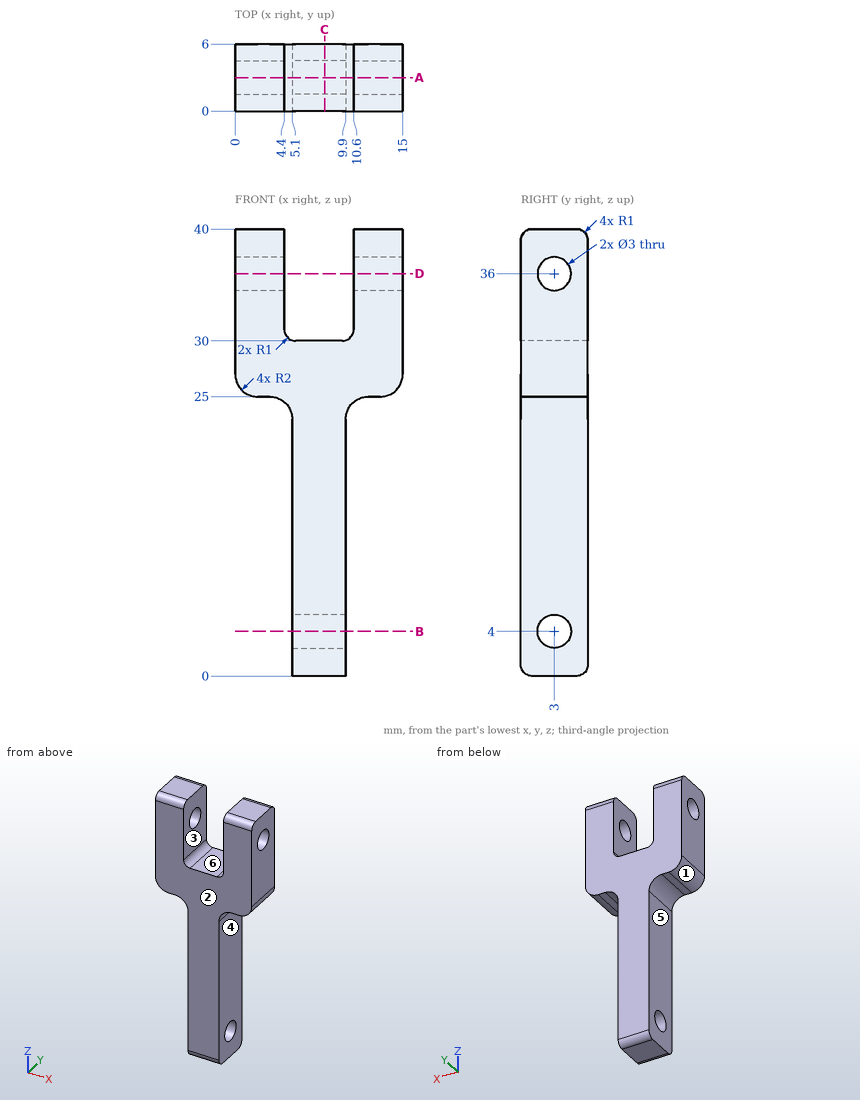
Can you work these out from the drawing? Everything is in mm from the part's minimum corner. A direction names the side the tool comes from. Give positions to 0.01 mm unless a question says otherwise; leave off trailing zeros. Order: outer loops, then holes, each group sorted by start corner. A loop starts at its lowest first (then second) coordinate and runs counter-clockwise, first axis right, second up. Notation, with made-up numbers: M -3.75,65 L 43.25,65 A27 cw 43.25,84 Z; hole C 59,-11 d9. An arc over 180 degrees is marked long. Use a Markdown table: item, result. Add a question column.
1. Suppose I cut it at C-C (x = 8). List the corners of the cut face in (y, z) for me.
2. I need wall thicknesses on probe 1 along Y at (x, z) = (13.95, 36); probe 2 along Z at (x, y) = (14.25, 2.4); probe 3 along X at (y, z) = (1.95, 5.5). Which ranges of each line are inside material? Lowest first, please. Write a range as from..to.
3. On a 3-axis mill with a long thin cutter (end or side, diameter ignored), from which of +Z, -Z, +X, -X, +Y, -Y can I reach the whole of each face in a straight line? I mean the marked faces 4, 5 and 6. Say none if no direction works.
4. Suppose I cut it at A-A (y = 3). Give the number of separate pieces and of enclosed holes in the cut face, and give its area (3 significant figures).
5. For pin 1 Ø3.5 at (y, z) = (3, 4) entering from +X; pin 2 Ø1.5 at (x, y) = (12, 0.5) entering from -Z; pin 3 Ø2.5 at (y, z) = (3, 36) entering from -X; pin 4 Ø1.2 at (x, y) = (12.5, 4.5) entering from -Z, each with a flat end and sliding along its axis, tell me the tip position at first contact or that it passes through.
6. If we mould it in two halves opening along X, with no side actions, what happens to the marked faces 1, 2 and 3? For each: +X half, -X half, draft (parallel to the pull), parting line (faces both ways), or undercut.
7. Suppose I cut it at D-D (z = 36). List the corners of the cut face in (x, y) for me.
8. Suppose I cut it at B-B (z = 4). List the corners of the cut face in (x, y) for me.
Results list:
| question | item | result |
|---|---|---|
| 1 | outline | M 0,1 A1 ccw 1,0 L 5,0 A1 ccw 6,1 L 6,30 L 0,30 Z; hole C 3,4 d3 |
| 2 | probe 1 | y = 0..1.5, 4.5..6 |
| 2 | probe 2 | z = 25.44..34.63, 37.37..40 |
| 2 | probe 3 | x = 5.1..9.9 |
| 3 | face 4 | -Z, +X, +Y, -Y |
| 3 | face 5 | -Z, -X, +Y, -Y |
| 3 | face 6 | +Z, +Y, -Y |
| 4 | separate pieces | 4 |
| 4 | enclosed holes | 0 |
| 4 | area | 243 mm² |
| 5 | pin 1 | stops at x = 9.9 |
| 5 | pin 2 | stops at z = 24.89 |
| 5 | pin 3 | passes through |
| 5 | pin 4 | stops at z = 25 |
| 6 | face 1 | -X half |
| 6 | face 2 | draft |
| 6 | face 3 | undercut |
| 7 | outline | M 0,0 L 4.4,0 L 4.4,1.5 L 0,1.5 Z; M 0,4.5 L 4.4,4.5 L 4.4,6 L 0,6 Z; M 10.6,0 L 15,0 L 15,1.5 L 10.6,1.5 Z; M 10.6,4.5 L 15,4.5 L 15,6 L 10.6,6 Z |
| 8 | outline | M 5.1,0 L 9.9,0 L 9.9,1.5 L 5.1,1.5 Z; M 5.1,4.5 L 9.9,4.5 L 9.9,6 L 5.1,6 Z |
